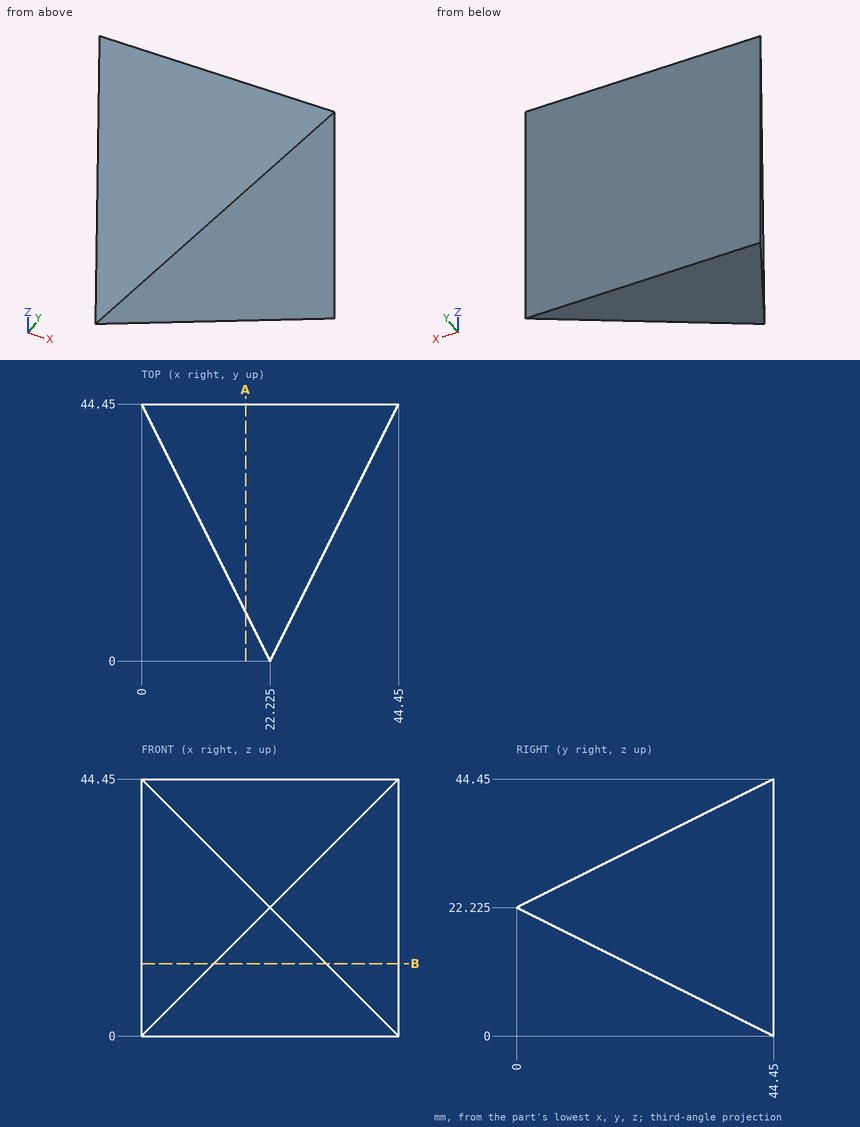
Design review of the part shown in the three views and the two pictorial views. Dimensions are in mm from the part's minimum x, y and z. Round coordinates to 2 decimals unless told otherwise and drop trailing zeros. Write each loop counter-clockwise with the first axis right and the second up, starting at its lowest first coordinate (ties: lowest second). Pieces come first, ordered by that corner, then holes.
Item 1: For pin 1 Ø6 at (y, z) = (24, 16.5) entering from -X (3 decimals); pin 2 Ø6 at (y, z) = (39.5, 25) entering from +X (3 decimals); pin 3 Ø10 at (x, y) = (31.5, 23.5) entering from -Z (3 decimals), all flat-tipped, find the tip position at first contact; note any pin that passes through.
Item 2: Wall thickness on L1, parallel to Y at x = 28, z = 19; L2, parallel to X at y = 10.5, z = 19 (3 decimals); L3, parallel to Y at x = 33, z = 20: over which ranges is each line inside the solid? List them lowest first.
Item 3: Consider section A-A on x = 18. Give the boundary of the cut face in (y, z), and give its area (3 significant figures).
Item 4: Consider section B-B on z = 12.5. Give the boundary of the cut face in (x, y), and give its area (3 significant figures).
Check values:
1. pin 1: stops at x = 8.725
1. pin 2: stops at x = 43.475
1. pin 3: stops at z = 7.975
2. L1: y = 11.55 to 44.45
2. L2: x = 16.975 to 27.475
2. L3: y = 21.55 to 44.45
3. outline: (8.45, 18) - (44.45, 0) - (44.45, 44.45) - (8.45, 26.45) - close
3. area: 952 mm2
4. outline: (0, 44.45) - (12.5, 19.45) - (31.95, 19.45) - (44.45, 44.45) - close
4. area: 799 mm2
